```python
from build123d import *

# Parameters (mm, degrees)
SKETCH1_W           = 276
SKETCH1_H           = 144
SKETCH1_R           = 2.5
BOSS_EXTRUDE1_DEPTH = 6.35
SKETCH2_R           = 2.5
CUT_EXTRUDE1_DEPTH  = 156.782933918
BOSS_EXTRUDE2_DEPTH = 6.35
SKETCH4_R           = 2.5
CUT_EXTRUDE2_DEPTH  = 163.727755776
FILLET1_R           = 3
SKETCH5_R           = 2.5
CUT_EXTRUDE3_DEPTH  = 163.727755776
SKETCH6_R           = 2.5
CUT_EXTRUDE4_DEPTH  = 163.727755776


with BuildPart() as part:
    # Sketch1 → Boss-Extrude1 (new body)
    with BuildSketch(Plane.XY):
        Rectangle(SKETCH1_W, SKETCH1_H)
        with Locations((-118, -66)):
            Circle(SKETCH1_R, mode=Mode.SUBTRACT)
        with Locations((-82, -66)):
            Circle(SKETCH1_R, mode=Mode.SUBTRACT)
        with Locations((-82, -34)):
            Circle(SKETCH1_R, mode=Mode.SUBTRACT)
        with Locations((-118, -34)):
            Circle(SKETCH1_R, mode=Mode.SUBTRACT)
        with Locations(Location((-118, 66, 0), (0, 0, 180))):
            Circle(SKETCH1_R, mode=Mode.SUBTRACT)
        with Locations(Location((-82, 66, 0), (0, 0, 180))):
            Circle(SKETCH1_R, mode=Mode.SUBTRACT)
        with Locations(Location((-82, 34, 0), (0, 0, 180))):
            Circle(SKETCH1_R, mode=Mode.SUBTRACT)
        with Locations(Location((-118, 34, 0), (0, 0, 180))):
            Circle(SKETCH1_R, mode=Mode.SUBTRACT)
        with Locations(Location((118, -66, 0), (0, 0, 180))):
            Circle(SKETCH1_R, mode=Mode.SUBTRACT)
        with Locations(Location((82, -66, 0), (0, 0, 180))):
            Circle(SKETCH1_R, mode=Mode.SUBTRACT)
        with Locations(Location((82, -34, 0), (0, 0, 180))):
            Circle(SKETCH1_R, mode=Mode.SUBTRACT)
        with Locations(Location((118, -34, 0), (0, 0, 180))):
            Circle(SKETCH1_R, mode=Mode.SUBTRACT)
        with Locations((118, 34)):
            Circle(SKETCH1_R, mode=Mode.SUBTRACT)
        with Locations((82, 34)):
            Circle(SKETCH1_R, mode=Mode.SUBTRACT)
        with Locations((82, 66)):
            Circle(SKETCH1_R, mode=Mode.SUBTRACT)
        with Locations((118, 66)):
            Circle(SKETCH1_R, mode=Mode.SUBTRACT)
    extrude(amount=BOSS_EXTRUDE1_DEPTH)

    # Sketch2 → Cut-Extrude1 (cut, through all)
    with BuildSketch(Plane.XY.offset(6.35)):
        with Locations((-66, -15)):
            Circle(SKETCH2_R)
        with Locations((-34, -15)):
            Circle(SKETCH2_R)
        with Locations(Location((-34, -51, 0), (0, 0, 180))):
            Circle(SKETCH2_R)
        with Locations(Location((-66, -51, 0), (0, 0, 180))):
            Circle(SKETCH2_R)
        with Locations((66, -51)):
            Circle(SKETCH2_R)
        with Locations((34, -51)):
            Circle(SKETCH2_R)
        with Locations(Location((34, -15, 0), (0, 0, 180))):
            Circle(SKETCH2_R)
        with Locations(Location((66, -15, 0), (0, 0, 180))):
            Circle(SKETCH2_R)
    extrude(amount=-CUT_EXTRUDE1_DEPTH, mode=Mode.SUBTRACT)

    # Sketch3 → Boss-Extrude2 (add, through all)
    with BuildSketch(Plane.XY.offset(6.35)):
        Polygon((-138, 72), (-124, 86), (124, 86), (138, 72), align=None)
    extrude(amount=-BOSS_EXTRUDE2_DEPTH)

    # Sketch4 → Cut-Extrude2 (cut, through all)
    with BuildSketch(Plane.XY.offset(6.35)):
        with Locations((-66, -15)):
            Circle(SKETCH4_R)
        with Locations((-34, -15)):
            Circle(SKETCH4_R)
        with Locations(Location((-34, -51, 0), (0, 0, 180))):
            Circle(SKETCH4_R)
        with Locations(Location((-66, -51, 0), (0, 0, 180))):
            Circle(SKETCH4_R)
        with Locations((-66, 29)):
            Circle(SKETCH4_R)
        with Locations((-66, 65)):
            Circle(SKETCH4_R)
        with Locations((-34, 65)):
            Circle(SKETCH4_R)
        with Locations((-34, 29)):
            Circle(SKETCH4_R)
        with Locations(Location((34, 29, 0), (0, 0, 180))):
            Circle(SKETCH4_R)
        with Locations(Location((34, 65, 0), (0, 0, 180))):
            Circle(SKETCH4_R)
        with Locations(Location((66, 65, 0), (0, 0, 180))):
            Circle(SKETCH4_R)
        with Locations(Location((66, 29, 0), (0, 0, 180))):
            Circle(SKETCH4_R)
        with Locations((34, -51)):
            Circle(SKETCH4_R)
        with Locations(Location((34, -15, 0), (0, 0, 180))):
            Circle(SKETCH4_R)
        with Locations(Location((66, -15, 0), (0, 0, 180))):
            Circle(SKETCH4_R)
        with Locations((66, -51)):
            Circle(SKETCH4_R)
    extrude(amount=-CUT_EXTRUDE2_DEPTH, mode=Mode.SUBTRACT)

    # Fillet1
    fillet1_edges = [part.edges().sort_by_distance(p)[0] for p in [
        (-124, 86, 3.175),
        (124, 86, 3.175),
        (138, -72, 3.175),
        (-138, -72, 3.175),
        (-138, 72, 3.175),
        (138, 72, 3.175),
    ]]
    fillet(fillet1_edges, radius=FILLET1_R)

    # Sketch5 → Cut-Extrude3 (cut, through all)
    with BuildSketch(Plane.XY.offset(6.35)):
        with Locations((-20, -32)):
            Circle(SKETCH5_R)
        with Locations(Location((20, -32, 0), (0, 0, 180))):
            Circle(SKETCH5_R)
        with Locations((20, -56)):
            Circle(SKETCH5_R)
        with Locations(Location((-20, -56, 0), (0, 0, 180))):
            Circle(SKETCH5_R)
    extrude(amount=-CUT_EXTRUDE3_DEPTH, mode=Mode.SUBTRACT)

    # Sketch6 → Cut-Extrude4 (cut, through all)
    with BuildSketch(Plane.XY.offset(6.35)):
        with Locations((12, 20)):
            Circle(SKETCH6_R)
        with Locations(Location((12, -20, 0), (0, 0, 180))):
            Circle(SKETCH6_R)
        with Locations((-12, -20)):
            Circle(SKETCH6_R)
        with Locations(Location((-12, 20, 0), (0, 0, 180))):
            Circle(SKETCH6_R)
    extrude(amount=-CUT_EXTRUDE4_DEPTH, mode=Mode.SUBTRACT)


solid = part.part
```
The listing builds one solid part. Answer for the finished solid, in the listing's coordinates (mm). Give positions to 0.01 mm unless a question says otherwise; leave off trailing zeros. Answer in a Markdown table with one row per item. Add a question column.
Q1. The part is cut by section A-A (z = 2). Give the number of separate pieces and of enclosed holes in the cut face, then the cut area to 3 significant figures.
Q2. Find the intervals of material crossed by line 1 along Y through (x, z) = (118, 3.75); line 2 along Y through (x, z) = (12, 2); line 3 along Y through (x, z) = (34, 2.5), in increasing order. Write a range as [from, to].
Q3. Given P1, Ø3, axis at x = -66, y = 65, coming from the +Z side, flat-ended and moving along its own axis, determine where the tip first touches the part or whether it passes through.
Q4. For a pull along X with two mould halves and no side action, classify faces 1 (the cylindrical face through (-32.66, 31.11, 3.22)), 2 (the flat face through (-138, 0, 3)), 3 (the flat face through (138, 0, 3)) as released by +X, released by -X, zero draft, split by the parting line, or undercut.
Determined:
| question | item | result |
|---|---|---|
| 1 | separate pieces | 1 |
| 1 | enclosed holes | 40 |
| 1 | area | 42,600 mm² |
| 2 | line 1 | y = [-72, -68.5], [-63.5, -36.5], [-31.5, 31.5], [36.5, 63.5], [68.5, 86] |
| 2 | line 2 | y = [-72, -22.5], [-17.5, 17.5], [22.5, 86] |
| 2 | line 3 | y = [-72, -53.5], [-48.5, -17.5], [-12.5, 26.5], [31.5, 62.5], [67.5, 86] |
| 3 | P1 | passes through |
| 4 | face 1 | undercut |
| 4 | face 2 | released by -X |
| 4 | face 3 | released by +X |
